from build123d import *

# Parameters (mm, degrees)
SKETCH1_W             = 141.2
SKETCH1_H             = 100
BOSS_EXTRUDE1_DEPTH   = 10
M4X0_7_TAPPED_HOLE1_D = 3.3


with BuildPart() as part:
    # Sketch1 → Boss-Extrude1 (new body)
    with BuildSketch(Plane.XY):
        with Locations((-70.6, 50)):
            Rectangle(SKETCH1_W, SKETCH1_H)
    extrude(amount=BOSS_EXTRUDE1_DEPTH)

    # M4x0.7 Tapped Hole1 (through all)
    with Locations(Plane.XY.offset(10)):
        with Locations((-120.6, 75), (-70.6, 50), (-95.6, 50), (-20.6, 50), (-45.6, 50), (-95.972807971, 50), (-120.6, 50), (-20.6, 25), (-45.6, 25), (-70.6, 25), (-95.6, 25), (-120.6, 25), (-20.6, 75), (-45.6, 75), (-70.6, 75), (-95.6, 75)):
            Hole(M4X0_7_TAPPED_HOLE1_D / 2)


solid = part.part
Model file for the job. Use its own axes, mm. Give positions to 0.01 mm unless a question says otherwise; leave off trailing zeros. Order: outer loops, then holes, each group sorted by start corner. A loop starts at its lowest first (then second) coordinate and runs counter-clockwise, first axis right, second up. Notation, with made-up numbers: (79, 72.25) - (125, 72.25) arc R11 cw to (125, 76.25) - close; hole circle Ø2 at (79, 74). An arc over 180 degrees is marked (long way). Return JSON: item names as keys, results as strings.
1) Cut at C-C, the plane y = 50. Give the cut face in (x, z), plus the area to 3 significant figures.
Geometry says:
{"outline": "(-141.2, 0) - (-122.25, 0) - (-122.25, 10) - (-141.2, 10) - close; (-118.95, 0) - (-97.62, 0) - (-97.62, 10) - (-118.95, 10) - close; (-93.95, 0) - (-72.25, 0) - (-72.25, 10) - (-93.95, 10) - close; (-68.95, 0) - (-47.25, 0) - (-47.25, 10) - (-68.95, 10) - close; (-43.95, 0) - (-22.25, 0) - (-22.25, 10) - (-43.95, 10) - close; (-18.95, 0) - (0, 0) - (0, 10) - (-18.95, 10) - close", "area": "1,240 mm²"}
2) Cut at A-A, the plane y = 25. Give the cut face in (x, z), plus the area to 3 significant figures.
Geometry says:
{"outline": "(-141.2, 0) - (-122.25, 0) - (-122.25, 10) - (-141.2, 10) - close; (-118.95, 0) - (-97.25, 0) - (-97.25, 10) - (-118.95, 10) - close; (-93.95, 0) - (-72.25, 0) - (-72.25, 10) - (-93.95, 10) - close; (-68.95, 0) - (-47.25, 0) - (-47.25, 10) - (-68.95, 10) - close; (-43.95, 0) - (-22.25, 0) - (-22.25, 10) - (-43.95, 10) - close; (-18.95, 0) - (0, 0) - (0, 10) - (-18.95, 10) - close", "area": "1,250 mm²"}
3) Probe line 1 (Y direction, x = -20.6, z = 4.75); line 2 (Y direction, x = -97, z = 5). List the from-to ranges inside material, lowest first. Write a range as from..to.
Geometry says:
{"line 1": "0..23.35, 26.65..48.35, 51.65..73.35, 76.65..100", "line 2": "0..24.13, 25.87..48.71, 51.29..74.13, 75.87..100"}
4) Pull direction Y, two halves, no side cores. Call faces 1 (the flat face through (-72, 100, 5)), 2 (the flat face through (-72, 62, 10)), 3 (the cylindrical face through (-119.384, 26.115, 4.93)): pulls with the +Y half, pulls with the -Y half, needs draft (parallel to the pull), parting line crosses it, or undercut.
Geometry says:
{"face 1": "pulls with the +Y half", "face 2": "needs draft", "face 3": "undercut"}
5) Flat gauge pin, fed straight in: P1, Ø4, axis at x = -70.6, y = 75, coming from the -Z side. Where does the tip first touch, or does it go through?
Geometry says:
{"P1": "z = 0"}
6) Cut at B-B, the plane x = -45.6. Give the cut face in (y, z).
Geometry says:
{"outline": "(0, 0) - (23.35, 0) - (23.35, 10) - (0, 10) - close; (26.65, 0) - (48.35, 0) - (48.35, 10) - (26.65, 10) - close; (51.65, 0) - (73.35, 0) - (73.35, 10) - (51.65, 10) - close; (76.65, 0) - (100, 0) - (100, 10) - (76.65, 10) - close"}
